Can you work these out from the model? Positions are in its coordinate system, mm. A direction names the side the tool comes from. Round coordinates to 2 decimals unless told otherwise and drop trailing zeros. Loops run counter-clockwise (first coordinate to the right, second up) from the corner with the lowest first, then second, coordinate; pieces in that order, holes last.
(1) I want a section at C-C on z = 43.25. Write out the boundary of the cut face in (x, y), plus the area to 3 significant figures.
(2) Will this pin go through, and if not, where does the flat tip stop? pin 1 Ø3.5 at (x, y) = (-71.25, -11.38) entering from +Z.
(3) If I drill on line 1 along Y through (x, z) = (-58, 40.25); line 2 along X through (y, z) = (-10.5, 38); line 3 along Z through (x, y) = (-59.75, -7.75), over which ranges is the centre line in solid material (lowest first)?
(4) I want a section at D-D on z = 41.5. Write out the boundary of the cut face in (x, y).
(5) I want a section at B-B on x = -70.75. Write out the boundary of the cut face in (y, z).
(6) Which directions (+Z, -Z, +X, -X, +Y, -Y) give clear straight access to the entire face, cutting with the end or side of a thin tool? Please do faces 4 (the face through (-69.31, -10.58, 42.07)), 5 (the face through (-60, -23.682, 42)).
(7) Thinking about a two-plate mould opening in Y: for faces 1 (the face through (-60, 3.118, 42)), 2 (the face through (-74.251, -11, 42)), 3 (the face through (-59.6, -11.2, 39.4)), which applies, released by +Y, released by -Y, zero draft, split by the parting line, or undercut?
(8) I want a section at A-A on z = 46.5. Write out the boundary of the cut face in (x, y), plus the area to 3 significant figures.
from build123d import *

# Parameters (mm, degrees)
SKETCH_W        = 29
SKETCH_H        = 29
SKETCH_R        = 2.1
PAD_DEPTH       = 10
SKETCH001_R     = 7.6
POCKET_DEPTH    = 35
SKETCH002_W     = 15.2
SKETCH002_H     = 2.2
PAD001_DEPTH    = 9
SKETCH003_R     = 4.638792
POCKET001_DEPTH = 35


with BuildPart() as part:
    # Sketch → Pad (new body)
    with BuildSketch(Plane(origin=(-33.3, -30, 47), x_dir=(1, 0, 0), z_dir=(0, 0, -1))):
        with Locations((-26.451358, -18.618412)):
            Rectangle(SKETCH_W, SKETCH_H)
        with Locations((-37.951358, -18.618412)):
            Circle(SKETCH_R, mode=Mode.SUBTRACT)
        with Locations((-14.951358, -18.618412)):
            Circle(SKETCH_R, mode=Mode.SUBTRACT)
    extrude(amount=PAD_DEPTH)

    # Sketch001 → Pocket (cut)
    with BuildSketch(Plane(origin=(-33.3, 3.118412, 47), x_dir=(1, 0, 0), z_dir=(0, 1, 0))):
        with Locations((-26.451358, 0)):
            Circle(SKETCH001_R)
    extrude(amount=-POCKET_DEPTH, mode=Mode.SUBTRACT)

    # Sketch002 → Pad001 (new body)
    with BuildSketch(Plane(origin=(-33.3, -30, 47), x_dir=(1, 0, 0), z_dir=(0, 0, 1))):
        with Locations((-26.451358, 32.018412)):
            Rectangle(SKETCH002_W, SKETCH002_H)
        with Locations((-26.451358, 5.218412)):
            Rectangle(SKETCH002_W, SKETCH002_H)
    extrude(amount=-PAD001_DEPTH)

    # Sketch003 → Pocket001 (cut)
    with BuildSketch(Plane(origin=(-33.3, -25.881588, 47), x_dir=(-1, 0, 0), z_dir=(0, -1, 0))):
        with Locations((26.451358, 0)):
            Circle(SKETCH003_R)
    extrude(amount=-POCKET001_DEPTH, mode=Mode.SUBTRACT)


solid = part.part
Filled sheet:
1. outline: (-74.25, -25.88) - (-62.48, -25.88) - (-62.48, -23.68) - (-66.36, -23.68) - (-66.36, 0.92) - (-62.48, 0.92) - (-62.48, 3.12) - (-74.25, 3.12) - close; (-57.02, -25.88) - (-45.25, -25.88) - (-45.25, 3.12) - (-57.02, 3.12) - (-57.02, 0.92) - (-53.14, 0.92) - (-53.14, -23.68) - (-57.02, -23.68) - close; hole circle Ø4.2 at (-71.25, -11.38); hole circle Ø4.2 at (-48.25, -11.38)
1. area: 464 mm2
2. pin 1: passes through
3. line 1: y = -25.88 to -23.68, 0.92 to 3.12
3. line 2: x = -74.25 to -73.16, -69.35 to -50.16, -46.35 to -45.25
3. line 3: z = 37 to 39.4
4. outline: (-74.25, -25.88) - (-45.25, -25.88) - (-45.25, 3.12) - (-74.25, 3.12) - close; hole circle Ø4.2 at (-71.25, -11.38); hole (-65, -23.68) - (-54.51, -23.68) - (-54.51, 0.92) - (-65, 0.92) - close; hole circle Ø4.2 at (-48.25, -11.38)
5. outline: (-25.88, 37) - (-13.42, 37) - (-13.42, 47) - (-25.88, 47) - close; (-9.34, 37) - (3.12, 37) - (3.12, 47) - (-9.34, 47) - close
6. face 4: +Z, -Z
6. face 5: +Z
7. face 1: released by +Y
7. face 2: zero draft
7. face 3: undercut
8. outline: (-74.25, -25.88) - (-64.36, -25.88) - (-64.36, -23.68) - (-67.33, -23.68) - (-67.33, 0.92) - (-64.36, 0.92) - (-64.36, 3.12) - (-74.25, 3.12) - close; (-55.14, -25.88) - (-45.25, -25.88) - (-45.25, 3.12) - (-55.14, 3.12) - (-55.14, 0.92) - (-52.17, 0.92) - (-52.17, -23.68) - (-55.14, -23.68) - close; hole circle Ø4.2 at (-71.25, -11.38); hole circle Ø4.2 at (-48.25, -11.38)
8. area: 400 mm2
